```python
from build123d import *

# Parameters (mm, degrees)
SKETCH1_R           = 63.5
BOSS_EXTRUDE1_DEPTH = 25.4
CHAMFER1_SIZE       = 10
SKETCH3_R           = 1.8161
CUT_EXTRUDE1_DEPTH  = 26.4


with BuildPart() as part:
    # Sketch1 → Boss-Extrude1 (new body)
    with BuildSketch(Plane.XY):
        with BuildLine():
            ThreePointArc((49.832360156, -73.620281725), (85.870805957, -23.00901311), (79.966230688, 38.84085413))
            ThreePointArc((79.966230688, 38.84085413), (82.48891971, 47.625), (73.620281725, 49.832360156))
            ThreePointArc((73.620281725, 49.832360156), (23.00901311, 85.870805957), (-38.84085413, 79.966230688))
            ThreePointArc((-38.84085413, 79.966230688), (-47.625, 82.48891971), (-49.832360156, 73.620281725))
            ThreePointArc((-49.832360156, 73.620281725), (-85.870805957, 23.00901311), (-79.966230688, -38.84085413))
            ThreePointArc((-79.966230688, -38.84085413), (-82.48891971, -47.625), (-73.620281725, -49.832360156))
            ThreePointArc((-73.620281725, -49.832360156), (-23.00901311, -85.870805957), (38.84085413, -79.966230688))
            ThreePointArc((38.84085413, -79.966230688), (47.625, -82.48891971), (49.832360156, -73.620281725))
        make_face()
        Circle(SKETCH1_R, mode=Mode.SUBTRACT)
    extrude(amount=BOSS_EXTRUDE1_DEPTH)

    # Chamfer1
    chamfer1_edges = [part.edges().sort_by_distance(p)[0] for p in [
        (-63.5, 0, 25.4),
    ]]
    chamfer(chamfer1_edges, length=CHAMFER1_SIZE)

    # Sketch3 → Cut-Extrude1 (cut, through all)
    with BuildSketch(Plane.XY.offset(25.4)):
        with Locations((74.789953871, 43.18)):
            Circle(SKETCH3_R)
        with Locations((43.18, -74.789953871)):
            Circle(SKETCH3_R)
        with Locations((-74.789953871, -43.18)):
            Circle(SKETCH3_R)
        with Locations((-43.18, 74.789953871)):
            Circle(SKETCH3_R)
    extrude(amount=-CUT_EXTRUDE1_DEPTH, mode=Mode.SUBTRACT)


solid = part.part
```
Geometry: final body of the model. Coordinates: model frame, mm. Give positions to 0.01 mm unless a question says otherwise; leave off trailing zeros. Loops run counter-clockwise (first coordinate to the right, second up) from the corner with the lowest first, then second, coordinate; pieces in that order, holes last. Notation, with made-up numbers: (-8, 30) -> (49, 30) arc R32 ccw to (49, 56) -> close; hole circle Ø4 at (30, -33.5). An arc over 180 degrees is marked (long way). Use one line per item in the form item = value.
Item 1: Section query B-B on z = 12.5. Output: boundary loops of the cut face in (x, y), and give its area (3 significant figures).
A:
outline = (-79.97, -38.84) arc R6.35 ccw (long way) to (-73.62, -49.83) arc R88.9 ccw to (38.84, -79.97) arc R6.35 ccw (long way) to (49.83, -73.62) arc R88.9 ccw to (79.97, 38.84) arc R6.35 ccw (long way) to (73.62, 49.83) arc R88.9 ccw to (-38.84, 79.97) arc R6.35 ccw (long way) to (-49.83, 73.62) arc R88.9 ccw to start; hole circle Ø3.63 at (-74.79, -43.18); hole circle Ø127 at (0, 0); hole circle Ø3.63 at (-43.18, 74.79); hole circle Ø3.63 at (43.18, -74.79); hole circle Ø3.63 at (74.79, 43.18)
area = 12,400 mm^2
Item 2: Line query: probe 1 along Y at (x, z) = (43.18, 12); probe 2 along Y at (x, z) = (-75, 8); probe 3 along X at (y, z) = (-23.5, 22.5). Output: solid intervals per line, ascending.
A:
probe_1 = -83.21 to -76.61, -72.97 to -46.56, 46.56 to 77.71
probe_2 = -50.48 to -44.98, -41.38 to 47.73
probe_3 = -85.74 to -66.57, 66.57 to 85.74
Item 3: Section query A-A on x = 0. Output: boundary loops of the cut face in (y, z), and give its area (3 significant figures).
A:
outline = (-88.9, 0) -> (-63.5, 0) -> (-63.5, 15.4) -> (-73.5, 25.4) -> (-88.9, 25.4) -> close; (63.5, 0) -> (88.9, 0) -> (88.9, 25.4) -> (73.5, 25.4) -> (63.5, 15.4) -> close
area = 1,190 mm^2
Item 4: Pin query (flat end, axial travel): P1, Ø6, axis at x = 28, z = 17.5, coming from the -Y side; P2, Ø8, axis at x = -30, z = 7.5, coming from the -Y side; P3, Ø12, axis at x = 52.5, z = 14.5, coming from the -Y side; P4, Ø3, axis at x = -43.18, y = 74.79, coming from the +Z side. Return the tip coordinate at first contact, or that it passes through.
A:
P1 = -85.31
P2 = -85.01
P3 = -83
P4 = through
